For this review, take the finished solid that the model builds, in its own axes (mm). Face numbers are marked on the shaded views. A direction names the side the tool comes from. Give positions to 0.01 mm unless a question says otherwise; leave off trailing zeros. Loops run counter-clockwise (first coordinate to the right, second up) from the corner with the lowest first, then second, coordinate; pieces in that order, holes last. Notation, with made-up numbers: (-4.5, -4.75) - (3.5, -4.75) arc R20 cw to (3.5, 2.25) - close; hole circle Ø2 at (4, 32.25). An arc over 180 degrees is marked (long way). Put each result on its own line as item: value. Start each with the question number.
from build123d import *

# Parameters (mm, degrees)
BASE_FLANGE1_DEPTH           = 30
EDGE_FLANGE1_STRIP_W         = 4.4196
EDGE_FLANGE1_STRIP_H         = 0.7366
EDGE_FLANGE1_STRIP_CUT_DEPTH = 45.5268
EDGE_FLANGE1_DEPTH           = 45.5268
M3_CLEARANCE_HOLE1_D         = 3.4
SKETCH13_R                   = 3
CUT_EXTRUDE2_DEPTH           = 52.675037868


# Sheet-metal steps are written as plain solids
with BuildPart() as part:
    # Sketch1 → Base-Flange1 (new, symmetric)
    with BuildSketch(Plane.XY):
        with BuildLine():
            Line((-23.5, 33), (-23.5, 0.7366))
            ThreePointArc((-23.5, 0.7366), (-23.284254855, 0.215745145), (-22.7634, 0))
            Line((-22.7634, 0), (22.7634, 0))
            ThreePointArc((22.7634, 0), (23.284254855, 0.215745145), (23.5, 0.7366))
            Line((23.5, 0.7366), (23.5, 33))
            Line((23.5, 33), (24.2366, 33))
            Line((24.2366, 33), (24.2366, 0.7366))
            ThreePointArc((24.2366, 0.7366), (23.80510971, -0.30510971), (22.7634, -0.7366))
            Line((22.7634, -0.7366), (-22.7634, -0.7366))
            ThreePointArc((-22.7634, -0.7366), (-23.80510971, -0.30510971), (-24.2366, 0.7366))
            Line((-24.2366, 0.7366), (-24.2366, 33))
            Line((-24.2366, 33), (-23.5, 33))
        make_face()
    extrude(amount=BASE_FLANGE1_DEPTH, both=True)

    # Edge-Flange1 strip (across the edge) → Edge-Flange1 strip cut (cut)
    with BuildSketch(Plane(origin=(-22.7634, 0, 30), x_dir=(0, 0, -1), z_dir=(1, 0, 0))):
        with Locations((-1.4732, -0.3683)):
            Rectangle(EDGE_FLANGE1_STRIP_W, EDGE_FLANGE1_STRIP_H)
    extrude(amount=EDGE_FLANGE1_STRIP_CUT_DEPTH, mode=Mode.SUBTRACT)

    # Edge-Flange1 section (across the edge) → Edge-Flange1 (add)
    with BuildSketch(Plane(origin=(-22.7634, 0, 30), x_dir=(0, 0, -1), z_dir=(1, 0, 0))):
        with BuildLine():
            Line((-0.7366, 0.7366), (-0.7366, 32.2634))
            Line((-0.7366, 32.2634), (0, 32.2634))
            Line((0, 32.2634), (0, 0.7366))
            ThreePointArc((0, 0.7366), (0.215745145, 0.215745145), (0.7366, 0))
            Line((0.7366, 0), (0.7366, -0.7366))
            ThreePointArc((0.7366, -0.7366), (-0.30510971, -0.30510971), (-0.7366, 0.7366))
        make_face()
    extrude(amount=EDGE_FLANGE1_DEPTH)

    # M3 Clearance Hole1 (through all)
    with Locations(Plane(origin=(24.2366, 0, 0), x_dir=(0, 0, -1), z_dir=(1, 0, 0))):
        with Locations((24, 22)):
            Hole(M3_CLEARANCE_HOLE1_D / 2)

    # Sketch13 → Cut-Extrude2 (cut, through all)
    with BuildSketch(Plane.XZ.offset(0.7366)):
        with Locations(Location((0, -6.5, 0), (0, 0, 270))):
            Circle(SKETCH13_R)
    extrude(amount=-CUT_EXTRUDE2_DEPTH, mode=Mode.SUBTRACT)


solid = part.part
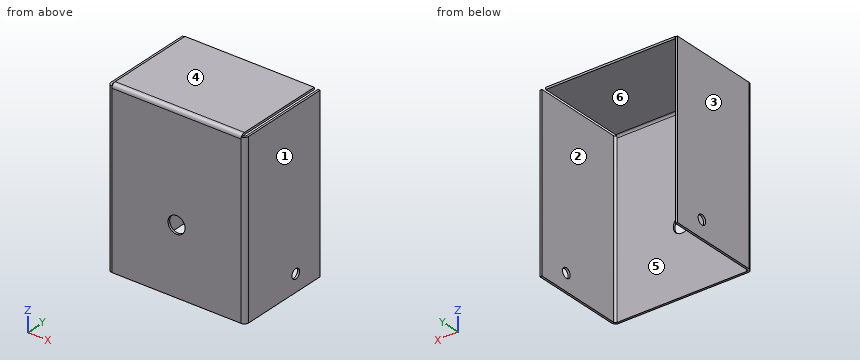
1) Take a section at C-C on x = -19. State the section outline as (y, z) points, and give its area (3 significant figures).
2) Mouldability with a two-part tool opening along X and no side actions: class the marked faces 3, 4, 5 and 6 as released by +X, released by -X, zero draft, split by the parting line, or undercut.
3) Take a section at B-B on z = -6.5. State the section outline as (x, y) points, and give its area (3 significant figures).
4) Wall thickness on probe 1 along X at (y, z) = (2.5, -13.5); probe 2 along Z at (x, y) = (14.5, 2); probe 3 along Y at (x, z) = (-3, 17): over which ranges is each line inside the solid? List them lowest first.
5) Insertion check: P1, Ø0.6, axis at x = 3.5, z = 30.5, coming from the +Y side; P2, Ø3.5, axis at x = 0, z = -6.5, coming from the +Y side; P3, Ø2, axis at x = -7, y = 16.5, coming from the -Z side; P4, Ø23, axis at x = -6, z = 4.5, coming from the +Y side. Each pin has a flat end and moves straight along its axis. Give the tip position at first contact, or say it passes through.
6) Take a section at D-D on x = 0. State the section outline as (y, z) points, and give its area (3 significant figures).
7) Take a section at A-A on y = 19.5. State the section outline as (x, z) points, and give its area (3 significant figures).
8) Machinability: for the marked faces 1 and 2, which of the approach directions +Z, -Z, +X, -X, +Y, -Y give a long, thin tool a straight path to every point of the face, cutting with its end or side? Answer none if there is none.
Answers follow:
1. outline: (-0.74, -30) - (0, -30) - (0, 29.26) arc R0.74 cw to (0.74, 30) - (32.26, 30) - (32.26, 30.74) - (0.74, 30.74) arc R1.47 ccw to (-0.74, 29.26) - close
1. area: 68.2 mm2
2. face 3: released by -X
2. face 4: zero draft
2. face 5: undercut
2. face 6: undercut
3. outline: (-24.24, 0.74) arc R1.47 ccw to (-22.76, -0.74) - (-3, -0.74) - (-3, 0) - (-22.76, 0) arc R0.74 cw to (-23.5, 0.74) - (-23.5, 33) - (-24.24, 33) - close; (3, -0.74) - (22.76, -0.74) arc R1.47 ccw to (24.24, 0.74) - (24.24, 33) - (23.5, 33) - (23.5, 0.74) arc R0.74 cw to (22.76, 0) - (3, 0) - close
3. area: 79.2 mm2
4. probe 1: -24.24 to -23.5, 23.5 to 24.24
4. probe 2: 30 to 30.74
4. probe 3: -0.74 to 0
5. P1: y = 32.26
5. P2: through
5. P3: z = 30
5. P4: y = 0
6. outline: (-0.74, -30) - (0, -30) - (0, -9.5) - (-0.74, -9.5) - close; (-0.74, -3.5) - (0, -3.5) - (0, 29.26) arc R0.74 cw to (0.74, 30) - (32.26, 30) - (32.26, 30.74) - (0.74, 30.74) arc R1.47 ccw to (-0.74, 29.26) - close
6. area: 63.7 mm2
7. outline: (-24.24, -30) - (-23.5, -30) - (-23.5, 30) - (-24.24, 30) - close; (-22.76, 30) - (22.76, 30) - (22.76, 30.74) - (-22.76, 30.74) - close; (23.5, -30) - (24.24, -30) - (24.24, 30) - (23.5, 30) - close
7. area: 122 mm2
8. face 1: +Z, -Z, +X, +Y, -Y
8. face 2: +Z, -Z, +Y
